For this review, take the finished solid that the model builds, in its own axes (mm). A direction names the side the tool comes from. Round coordinates to 2 decimals unless told otherwise and drop trailing zeros. Order: outer loops, then holes, each group sorted by start corner. A loop starts at its lowest first (then second) coordinate and runs counter-clockwise, first axis right, second up. Notation, with made-up numbers: M 41,70.25 L 61,70.25 A10 ccw 61,74.25 Z; hole C 42.5,83 d8. An arc over 180 degrees is marked long. Write item = value, one per line. Start each with the question number.
from build123d import *

# Parameters (mm, degrees)
SKETCH_1_R          = 1.5
EXTRUDE_1_DEPTH     = 6
SKETCH_2_W          = 106
SKETCH_2_H          = 60
EXTRUDE_2_DEPTH     = 46
SKETCH_3_R          = 2.913601035
SKETCH_3_W          = 27.829913336
SKETCH_3_H          = 14.266598172
SKETCH_3_W_2        = 28.231789341
SKETCH_3_W_3        = 5.927671071
SKETCH_3_H_2        = 3.014070036
SKETCH_3_W_4        = 6.731423082
SKETCH_3_H_3        = 3.918291047
CUT_EXTRUDE_1_DEPTH = 2
SKETCH_4_W          = 5.850937101
SKETCH_4_H          = 3.132319863
SKETCH_4_W_2        = 5.791836726
CUT_EXTRUDE_2_DEPTH = 10
SKETCH_5_W          = 25.590462272
SKETCH_5_H          = 8.924156589
CUT_EXTRUDE_3_DEPTH = 10


with BuildPart() as part:
    # 草图1 → 凸台-拉伸1 (new body)
    with BuildSketch(Plane(origin=(0, 0, 0), x_dir=(1, 0, 0), z_dir=(0, 1, 0))):
        Polygon((44.601753779, -30), (-44.601753779, -30), (-51.423054046, -39.075905643), (-60.615391847, -35.138784137), (-55.25, -28), (-55.25, -20), (-63.25, -20), (-63.25, 20), (-55.25, 20), (-55.25, 28), (-60.615391847, 35.138784137), (-51.423054046, 39.075905643), (-44.601753779, 30), (44.601753779, 30), (51.423054046, 39.075905643), (60.615391847, 35.138784137), (55.25, 28), (55.25, 20), (63.25, 20), (63.25, -20), (55.25, -20), (55.25, -28), (60.615391847, -35.138784137), (51.423054046, -39.075905643), align=None)
        with Locations(Location((58.25, 15, 0), (0, 0, 270))):
            Circle(SKETCH_1_R, mode=Mode.SUBTRACT)
        with Locations(Location((-58.25, 15, 0), (0, 0, 270))):
            Circle(SKETCH_1_R, mode=Mode.SUBTRACT)
        with Locations(Location((58.25, 9, 0), (0, 0, 270))):
            Circle(SKETCH_1_R, mode=Mode.SUBTRACT)
        with Locations(Location((-58.25, 9, 0), (0, 0, 270))):
            Circle(SKETCH_1_R, mode=Mode.SUBTRACT)
        with Locations(Location((58.25, -9, 0), (0, 0, 90))):
            Circle(SKETCH_1_R, mode=Mode.SUBTRACT)
        with Locations(Location((58.25, -15, 0), (0, 0, 90))):
            Circle(SKETCH_1_R, mode=Mode.SUBTRACT)
        with Locations(Location((-58.25, -9, 0), (0, 0, 90))):
            Circle(SKETCH_1_R, mode=Mode.SUBTRACT)
        with Locations(Location((-58.25, -15, 0), (0, 0, 90))):
            Circle(SKETCH_1_R, mode=Mode.SUBTRACT)
    extrude(amount=EXTRUDE_1_DEPTH)

    # 草图2 → 凸台-拉伸2 (add)
    with BuildSketch(Plane(origin=(0, 6, 0), x_dir=(1, 0, 0), z_dir=(0, 1, 0))):
        Rectangle(SKETCH_2_W, SKETCH_2_H)
    extrude(amount=EXTRUDE_2_DEPTH)

    # 草图3 → 切除-拉伸1 (cut)
    with BuildSketch(Plane(origin=(0, 0, -30), x_dir=(-1, 0, 0), z_dir=(0, 0, -1))):
        with Locations((7.233768087, 14.983525058)):
            Circle(SKETCH_3_R)
        with Locations((-28.282023842, 32.56560027)):
            Rectangle(SKETCH_3_W, SKETCH_3_H)
        with Locations((1.858676522, 32.56560027)):
            Rectangle(SKETCH_3_W_2, SKETCH_3_H)
        with Locations((-33.305473902, 14.481180052)):
            Rectangle(SKETCH_3_W_3, SKETCH_3_H_2)
        with Locations((-22.856697776, 14.029069547)):
            Rectangle(SKETCH_3_W_4, SKETCH_3_H_3)
        with Locations((-11.001355633, 14.029069547)):
            Rectangle(SKETCH_3_W_4, SKETCH_3_H_3)
    extrude(amount=-CUT_EXTRUDE_1_DEPTH, mode=Mode.SUBTRACT)

    # 草图4 → 切除-拉伸2 (cut)
    with BuildSketch(Plane(origin=(53, 0, 0), x_dir=(0, 0, -1), z_dir=(1, 0, 0))):
        with BuildLine():
            ThreePointArc((15.636259672, 23.370033323), (9.101457713, 29.904835281), (2.566655755, 23.370033323))
            Line((2.566655755, 23.370033323), (15.636259672, 23.370033323))
        make_face()
        with BuildLine():
            Line((15.636259672, 23.370033323), (2.566655755, 23.370033323))
            ThreePointArc((2.566655755, 23.370033323), (9.101457713, 16.835231365), (15.636259672, 23.370033323))
        make_face()
        with BuildLine():
            ThreePointArc((15.636259672, 23.370033323), (9.101457713, 16.835231365), (2.566655755, 23.370033323))
            Line((2.566655755, 23.370033323), (2.566655755, 7.058329889))
            Line((2.566655755, 7.058329889), (15.636259672, 7.058329889))
            Line((15.636259672, 7.058329889), (15.636259672, 23.370033323))
        make_face()
        with Locations((-9.3674094, 36.992669706)):
            Rectangle(SKETCH_4_W, SKETCH_4_H)
        with Locations((-17.789212803, 36.992669706)):
            Rectangle(SKETCH_4_W_2, SKETCH_4_H)
    extrude(amount=-CUT_EXTRUDE_2_DEPTH, mode=Mode.SUBTRACT)

    # 草图5 → 切除-拉伸3 (cut)
    with BuildSketch(Plane.ZY.offset(53)):
        with BuildLine():
            Line((10.519866707, 31.703186164), (10.519866707, 15.155081231))
            ThreePointArc((10.519866707, 15.155081231), (17.316409805, 21.951624329), (24.112952903, 15.155081231))
            Line((24.112952903, 15.155081231), (24.112952903, 31.703186164))
            Line((24.112952903, 31.703186164), (10.519866707, 31.703186164))
        make_face()
        with BuildLine():
            ThreePointArc((24.112952903, 15.155081231), (17.316409805, 21.951624329), (10.519866707, 15.155081231))
            Line((10.519866707, 15.155081231), (24.112952903, 15.155081231))
        make_face()
        with BuildLine():
            Line((24.112952903, 15.155081231), (10.519866707, 15.155081231))
            ThreePointArc((10.519866707, 15.155081231), (17.316409805, 8.358538134), (24.112952903, 15.155081231))
        make_face()
        with Locations((-5.821386914, 36.165264459)):
            Rectangle(SKETCH_5_W, SKETCH_5_H)
    extrude(amount=-CUT_EXTRUDE_3_DEPTH, mode=Mode.SUBTRACT)


solid = part.part
(1) We need section C-C, the plane z = -33.5. Write out the cut boundary in (x, y), then the cut area to 3 significant figures.
(2) Draft analysis for pull direction Z (two halves, no side actions). For faces 1 (the flat face through (-1, 20, -30)), 2 (the flat face through (48, 35.427, 18)), 3 (the cylindrical face through (-4.92, 13.21, -29.01)), 4 (the flat face through (59, 3, -20)), state which applies: released by +Z, released by -Z, zero draft, split by the parting line, or undercut.
(3) For faces 5 (the flat face through (53, 29, 0)), 6 (the flat face through (48, 37, 20.685)), 7 (the cylindrical face through (-48.07, 8.36, 17.17)), 8 (the flat face through (57.895, 2.958, 31.519)), list the 3-axis set-ups (+Z, -Z, +X, -X, +Y, -Y) from which the entire face can be reached by the end or side of a thin tool; tool diameter is ignored.
(4) We need section B-B, the plane x = 35. Write out the cut boundary in (y, z), then the cut area to 3 significant figures.
(5) Insertion check: pin 1 (2 mm diameter, centred on y = 44, z = 2.5, fed in from +X); pin 2 (1 mm diameter, centred on y = 46, z = -20, fed in from -X); pin 3 (7 mm diameter, centred on x = -50, y = 36, fed in from +Z); pin 4 (2.5 mm diameter, centred on x = 58.25, z = 15, fed in from -Y). Each pin has a flat end and moves straight along its axis. Give the tip position at first contact, or say it passes through.
(6) We need section D-D, the plane x = 58.25. Write out the cut boundary in (y, z), then the cut area to 3 significant figures.
(7) We need section A-A, the plane z = 9. Write out the cut boundary in (x, y).
(8) For line 1 along X through (y, z) = (3.3, -15); line 2 along Y through (x, z) = (-44, -12.5); line 3 along Z through (x, y) = (38.5, 9), list the stretches that pass through material, from the lowest coordinate up.
Values:
q1.outline = M -59.38,0 L -47.23,0 L -47.23,6 L -59.38,6 Z; M 47.23,0 L 59.38,0 L 59.38,6 L 47.23,6 Z
q1.area = 146 mm²
q2.face_1 = released by -Z
q2.face_2 = undercut
q2.face_3 = zero draft
q2.face_4 = undercut
q3.face_5 = +Z, -Z, +X, +Y
q3.face_6 = +X
q3.face_7 = -X
q3.face_8 = +X, +Y, -Y
q4.outline = M 0,-30 L 12.97,-30 L 12.97,-28 L 15.99,-28 L 15.99,-30 L 25.43,-30 L 25.43,-28 L 39.7,-28 L 39.7,-30 L 52,-30 L 52,30 L 0,30 Z
q4.area = 3,090 mm²
q5.pin_1 = 53
q5.pin_2 = -53
q5.pin_3 = 30
q5.pin_4 = through
q6.outline = M 0,-36.15 L 6,-36.15 L 6,-31.99 L 0,-31.99 Z; M 0,-20 L 6,-20 L 6,-16.5 L 0,-16.5 Z; M 0,-13.5 L 6,-13.5 L 6,-10.5 L 0,-10.5 Z; M 0,-7.5 L 6,-7.5 L 6,7.5 L 0,7.5 Z; M 0,10.5 L 6,10.5 L 6,13.5 L 0,13.5 Z; M 0,16.5 L 6,16.5 L 6,20 L 0,20 Z; M 0,31.99 L 6,31.99 L 6,36.15 L 0,36.15 Z
q6.area = 218 mm²
q7.outline = M -63.25,0 L -59.75,0 L -59.75,6 L -63.25,6 Z; M -56.75,0 L 56.75,0 L 56.75,6 L 53,6 L 53,35.43 L 43,35.43 L 43,38.56 L 53,38.56 L 53,52 L -53,52 L -53,6 L -56.75,6 Z; M 59.75,0 L 63.25,0 L 63.25,6 L 59.75,6 Z
q8.line_1 = -63.25 to -59.75, -56.75 to 56.75, 59.75 to 63.25
q8.line_2 = 0 to 31.7, 40.63 to 52
q8.line_3 = -30 to 30
